```python
from build123d import *

# Parameters (mm, degrees)
F0_W      = 39.9796
F0_H      = 39.968465
F1_DEPTH  = 40.0304
F2_R      = 16.341879
F2_R_2    = 11.603864
F3_DEPTH  = 70.612
F4_W      = 39.9796
F4_H      = 39.9796
F5_DEPTH  = 39.9796
F6_R      = 17.778332
F7_DEPTH  = 74.93
F8_W      = 39.895397
F8_H      = 39.822329
F8_H_2    = 39.968465
F9_DEPTH  = 49.276
F10_R     = 7.86972
F11_DEPTH = 116.332


with BuildPart() as f1:
    # F0 (on Top) → F1 (new body)
    with BuildSketch(Plane.XY):
        with Locations((19.9898, 19.984232)):
            Rectangle(F0_W, F0_H)
    extrude(amount=F1_DEPTH)

    # F2 (on Top) → F3 (join)
    with BuildSketch(Plane.XY):
        with Locations((20.166904, 19.655425)):
            Circle(F2_R)
        with Locations((20.166904, 19.655425)):
            Circle(F2_R_2, mode=Mode.SUBTRACT)
    extrude(amount=F3_DEPTH)

    # F4 (on Top) → F5 (join)
    with BuildSketch(Plane.XY):
        with Locations((19.9898, -19.9898)):
            Rectangle(F4_W, F4_H)
    extrude(amount=F5_DEPTH)

    # F6 (on Top) → F7 (join)
    with BuildSketch(Plane.XY):
        with Locations((19.436218, -20.678384)):
            Circle(F6_R)
    extrude(amount=F7_DEPTH)

    # F8 (on Top) → F9 (join)
    with BuildSketch(Plane.XY):
        with Locations((19.947698, 19.911164)):
            Rectangle(F8_W, F8_H)
        with Locations((19.947698, -19.984232)):
            Rectangle(F8_W, F8_H_2)
    extrude(amount=F9_DEPTH)

    # F10 (on Top) → F11 (join)
    with BuildSketch(Plane.XY):
        with Locations((19.290084, -21.847481)):
            Circle(F10_R)
    extrude(amount=F11_DEPTH)


solid = f1.part
```
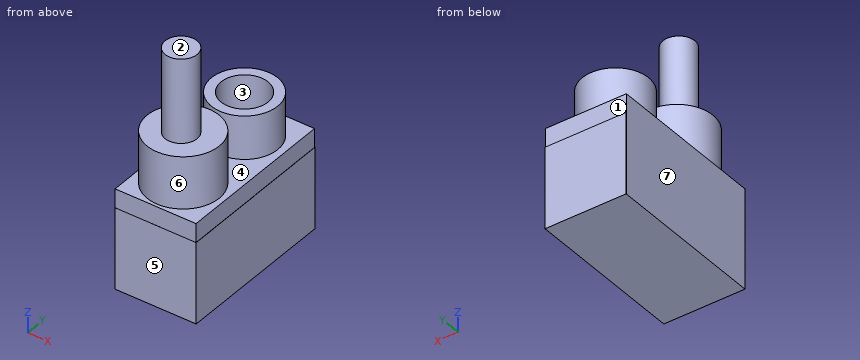
Geometry: final body of the model. Coordinates: model frame, mm. Face numbers are marked on the shaded views. A direction names the side the tool comes from. Coordinates: 2 decimals unless noted, no trailing zeros. Order: outer loops, then holes, each group sorted by start corner. A loop starts at its lowest first (then second) coordinate and runs counter-clockwise, first axis right, second up.
Item 1: Draft query along Y for the marked faces 4, 5, 6 and 7. Return one class per face: released by +Y, released by -Y, zero draft, split by the parting line, or undercut.
Answer:
face 4: undercut
face 5: released by -Y
face 6: undercut
face 7: zero draft
Item 2: Contact query for flat-ended pins moving along their axis: P1, Ø10, axis at x = 28, y = -28.5, coming from the -Z side; P2, Ø18.5, axis at x = 20.17, y = 19.66, coming from the +Z side; P3, Ø12, axis at x = 32, z = 70, coming from the +Y side; P4, Ø1.5, axis at x = 28.5, y = 12.5, coming from the +Z side. Output: stop coordinate, or through.
Answer:
P1: stops at z = 0
P2: stops at z = 49.28
P3: stops at y = 34.92
P4: stops at z = 70.61
Item 3: Section query D-D (z = 105). Output: boundary loops of the cut face in (x, y), then the cut area to 3 significant figures.
Answer:
outline: circle Ø15.74 at (19.29, -21.85)
area: 195 mm2
Item 4: Section query C-C (z = 52). Output: boundary loops of the cut face in (x, y), then the cut area to 3 significant figures.
Answer:
outline: circle Ø35.56 at (19.44, -20.68); circle Ø32.68 at (20.17, 19.66); hole circle Ø23.21 at (20.17, 19.66)
area: 1,410 mm2
Item 5: Section query B-B (y = 9.5). Output: boundary loops of the cut face in (x, z), then the cut area to 3 significant figures.
Answer:
outline: (0, 0) - (39.98, 0) - (39.98, 40.03) - (39.9, 40.03) - (39.9, 49.28) - (32.97, 49.28) - (32.97, 70.61) - (25.78, 70.61) - (25.78, 49.28) - (14.55, 49.28) - (14.55, 70.61) - (7.36, 70.61) - (7.36, 49.28) - (0, 49.28) - close
area: 2,280 mm2
Item 6: Material intervals for line 1 along Y through (x, z) = (28, 64); line 2 along Z through (x, y) = (11.5, 36.5); line 3 along Z through (x, y) = (15.5, -35.5), sorted ascending.
Answer:
line 1: y = -36.26 to -5.1, 5.31 to 11.09, 28.22 to 34
line 2: z = 0 to 49.28
line 3: z = 0 to 74.93
Item 7: Access query for the marked faces 1, 2 and 3. Directions: +Z, -Z, +X, -X, +Y, -Y. A direction counts if a zero-diameter tool reaches every point of the face in a straight line with its end or side. Return the directions, or none.
Answer:
face 1: +Z, +X, -X, +Y
face 2: +Z, +X, -X, +Y, -Y
face 3: +Z
